Source: CAD feature listing. Evaluate the final solid. Frame: model axes, mm. Face numbers are marked on the shaded views. A direction names the side the tool comes from. Give positions to 0.01 mm unless a question says otherwise; leave off trailing zeros. Order: outer loops, then holes, each group sorted by start corner. A loop starts at its lowest first (then second) coordinate and runs counter-clockwise, first axis right, second up. Notation, with made-up numbers: M 52,-9.5 L 96,-9.5 A12 ccw 96,-4.5 Z; hole C 61.25,-5.5 d2. An arc over 180 degrees is marked long. Use CSV: the item, a comma, the result in double quotes. Start each with the question number.
Item 1: First-contact query: pin 1 (11 mm diameter, centred on x = -11.5, y = -11, fed in from -Z); pin 2 (1 mm diameter, centred on x = -18, y = 3, fed in from -Z); pin 3 (4 mm diameter, centred on x = 5, y = -12.5, fed in from -Z); pin 4 (3 mm diameter, centred on x = -2.5, y = -11, fed in from -Z). Flat tips, straight axial feed; report the tip coordinate or a pass-through.
Item 2: Access query for the marked faces 5 and 6. Directions: +Z, -Z, +X, -X, +Y, -Y. A direction counts if a zero-diameter tool reaches every point of the face in a straight line with its end or side. Return the directions, or none.
Item 3: Section query B-B on x = 8.5. Return loops of the section in (y, z), and give its area (3 significant figures).
Item 4: Ray query, probe 1 along X at (y, z) = (-15.75, 6); probe 2 along X at (y, z) = (-3.25, 4.25); probe 3 along Y at (x, z) = (-0.5, 2). Return the intervals inside material, ascending. Write a range as from..to.
Item 5: Section query C-C on z = 6.5. Return loops of the section in (x, y).
Item 6: Pull-direction query (X, two-part tool) for the marked faces 1, 2, 3 and 4; classes: +X half, -X half, draft (parallel to the pull), parting line (faces both ways), or undercut.
Item 7: Section query D-D on y = -1. Return loops of the section in (x, z).
Item 8: Section query A-A on z = 1.25. Return loops of the section in (x, y), and give its area (3 significant figures).
from build123d import *

# Parameters (mm, degrees)
F0_W     = 40
F0_H     = 30
F0_W_2   = 14
F0_H_2   = 22
F0_R     = 4.2582963086
F0_W_3   = 4
F1_DEPTH = 15
F2_DEPTH = 8
F3_DEPTH = 4.4
F4_DEPTH = 4.3


with BuildPart() as f1:
    # F0 (on Top) → F1 (new body)
    with BuildSketch(Plane.XY):
        with Locations((-2.458587151, -7.6971892889)):
            Rectangle(F0_W, F0_H)
        Polygon((-18.458587151, -18.6971892889), (-18.458587151, 3.3028107111), (-4.458587151, 3.3028107111), (-0.458587151, 3.3028107111), (13.541412849, 3.3028107111), (13.541412849, -18.6971892889), (-0.458587151, -18.6971892889), (-4.458587151, -18.6971892889), align=None, mode=Mode.SUBTRACT)
        with Locations((-11.458587151, -7.6971892889)):
            Rectangle(F0_W_2, F0_H_2)
        with Locations((-11.3728679717, -7.7874381095)):
            Circle(F0_R, mode=Mode.SUBTRACT)
        with Locations((6.541412849, -7.6971892889)):
            Rectangle(F0_W_2, F0_H_2)
        with Locations((-2.458587151, -7.6971892889)):
            Rectangle(F0_W_3, F0_H_2)
        with Locations((-11.3728679717, -7.7874381095)):
            Circle(F0_R)
    extrude(amount=F1_DEPTH)

    # F0 (on Top) → F2 (cut)
    with BuildSketch(Plane.XY):
        with Locations((6.541412849, -7.6971892889)):
            Rectangle(F0_W_2, F0_H_2)
        with Locations((-11.458587151, -7.6971892889)):
            Rectangle(F0_W_2, F0_H_2)
        with Locations((-11.3728679717, -7.7874381095)):
            Circle(F0_R, mode=Mode.SUBTRACT)
    extrude(amount=F2_DEPTH, mode=Mode.SUBTRACT)

    # F0 (on Top) → F3 (cut)
    with BuildSketch(Plane.XY):
        with Locations((-11.3728679717, -7.7874381095)):
            Circle(F0_R)
    extrude(amount=F3_DEPTH, mode=Mode.SUBTRACT)

    # F0 (on Top) → F4 (cut)
    with BuildSketch(Plane.XY):
        with Locations((-2.458587151, -7.6971892889)):
            Rectangle(F0_W_3, F0_H_2)
    extrude(amount=F4_DEPTH, mode=Mode.SUBTRACT)


solid = f1.part
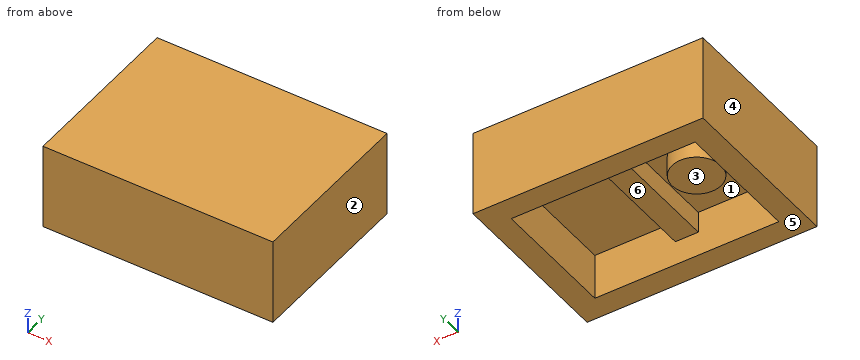
Verdict:
1,pin 1,"z = 4.4"
1,pin 2,"z = 0"
1,pin 3,"z = 8"
1,pin 4,"z = 4.3"
2,face 5,"-Z, +X, -X, +Y, -Y"
2,face 6,"-Z"
3,outline,"M -22.7,0 L -18.7,0 L -18.7,8 L 3.3,8 L 3.3,0 L 7.3,0 L 7.3,15 L -22.7,15 Z"
3,area,"274 mm2"
4,probe 1,"-22.46..-18.46, -4.46..-0.46, 13.54..17.54"
4,probe 2,"-22.46..-18.46, 13.54..17.54"
4,probe 3,"-22.7..-18.7, 3.3..7.3"
5,outline,"M -22.46,-22.7 L 17.54,-22.7 L 17.54,7.3 L -22.46,7.3 Z; C -11.37,-7.79 d8.52; hole M -18.46,-18.7 L -4.46,-18.7 L -4.46,3.3 L -18.46,3.3 Z; hole M -0.46,-18.7 L 13.54,-18.7 L 13.54,3.3 L -0.46,3.3 Z"
6,face 1,"undercut"
6,face 2,"+X half"
6,face 3,"undercut"
6,face 4,"-X half"
7,outline,"M -22.46,0 L -18.46,0 L -18.46,8 L -4.46,8 L -4.46,4.3 L -0.46,4.3 L -0.46,8 L 13.54,8 L 13.54,0 L 17.54,0 L 17.54,15 L -22.46,15 Z"
8,outline,"M -22.46,-22.7 L 17.54,-22.7 L 17.54,7.3 L -22.46,7.3 Z; hole M -18.46,-18.7 L 13.54,-18.7 L 13.54,3.3 L -18.46,3.3 Z"
8,area,"496 mm2"
